Design review of the part built by this model. Coordinates are the model's own, in mm. A direction names the side the tool comes from. Coordinates: 2 decimals unless noted, no trailing zeros. Loops run counter-clockwise (first coordinate to the right, second up) from the corner with the lowest first, then second, coordinate; pieces in that order, holes last. Notation, with made-up numbers: M 34,61.5 L 85,61.5 A31 ccw 85,87.5 Z; hole C 27,0.5 d4. An arc over 180 degrees is marked long. One line per item, written item: value.
```python
from build123d import *

# Parameters (mm, degrees)
SKETCH1_W           = 220
SKETCH1_H           = 39
BOSS_EXTRUDE1_DEPTH = 3
SKETCH2_W           = 155
SKETCH2_H           = 8
SKETCH2_W_2         = 80
SKETCH2_H_2         = 3
SKETCH2_R           = 1.5
CUT_EXTRUDE2_DEPTH  = 3


with BuildPart() as part:
    # Sketch1 → Boss-Extrude1 (new body)
    with BuildSketch(Plane(origin=(0, 0, 0), x_dir=(1, 0, 0), z_dir=(0, 1, 0))):
        Rectangle(SKETCH1_W, SKETCH1_H)
    extrude(amount=BOSS_EXTRUDE1_DEPTH)

    # Sketch2 → Cut-Extrude2 (cut)
    with BuildSketch(Plane.XZ):
        Polygon((-77, 16.5), (-80, 16.5), (-80, 13.5), (-81.25, 13.5), (-81.25, 10.5), (-80, 10.5), (-80, 8.5), (-77, 8.5), (-77, 10.5), (-75.75, 10.5), (-75.75, 13.5), (-77, 13.5), align=None)
        Polygon((-110, 16.5), (-80, 16.5), (-77, 16.5), (-70, 16.5), (-70, 19.5), (-110, 19.5), align=None)
        with Locations((-17.5, -15.5)):
            Rectangle(SKETCH2_W, SKETCH2_H)
        Polygon((110, 19.5), (75, 19.5), (75, 16.5), (75, -13), (75, -19.5), (110, -19.5), align=None)
        Polygon((75, 16.5), (75, 19.5), (30, 19.5), (30, 16.5), (37, 16.5), (40, 16.5), align=None)
        Polygon((40, 13.5), (40, 16.5), (37, 16.5), (37, 13.5), (35.75, 13.5), (35.75, 10.5), (37, 10.5), (37, 8.5), (40, 8.5), (40, 10.5), (41.25, 10.5), (41.25, 13.5), align=None)
        with Locations((-20, 18)):
            Rectangle(SKETCH2_W_2, SKETCH2_H_2)
        with Locations(Location((-102.5, -17, 0), (0, 0, 270))):
            Circle(SKETCH2_R)
        with Locations(Location((67.5, -17, 0), (0, 0, 270))):
            Circle(SKETCH2_R)
    extrude(amount=-CUT_EXTRUDE2_DEPTH, mode=Mode.SUBTRACT)


solid = part.part
```
(1) Tool access review of faces 1 (the flat face through (-19, 1, -11.5)), 2 (the flat face through (30, 1, 18)), 3 (the flat face through (-81.25, 1, 12)), 4 (the flat face through (40, 1, 15)), 5 (the flat face through (-70, 1, 18)): name each direction out of +Z, -Z, +X, -X, +Y, -Y from which nothing blocks a thin tool from reaching the whole face with its end or side.
Reply:
face 1: -Z, +Y, -Y
face 2: +Z, +X, +Y, -Y
face 3: +Y, -Y
face 4: +Z, +Y, -Y
face 5: +Z, -X, +Y, -Y
(2) Insertion check: pin 1 (1.4 mm diameter, centred on x = -80.5, y = 1.5, fed in from -Z); pin 2 (0.6 mm diameter, centred on x = -76, y = 1.5, fed in from +Z). Each pin has a flat end and moves straight along its axis. Give the tip position at first contact, or say it passes through.
Reply:
pin 1: stops at z = -11.5
pin 2: stops at z = 16.5
(3) We need section B-B on x = -9. State the section outline as (y, z) points, then the cut area to 3 significant figures.
Reply:
outline: M 0,-11.5 L 3,-11.5 L 3,16.5 L 0,16.5 Z
area: 84.0 mm2
(4) To check wall thickness, follow line 1 along X through (y, z) = (1.3, -17); line 2 along X through (y, z) = (2.8, 11.5); line 3 along Z through (x, y) = (-102.5, 0.85). State the ranges of each line that lie inside material, in increasing order. Write a range as [from, to].
Reply:
line 1: x = [-110, -104], [-101, -95], [60, 66], [69, 75]
line 2: x = [-110, -81.25], [-75.75, 35.75], [41.25, 75]
line 3: z = [-19.5, -18.5], [-15.5, 16.5]
(5) We need section A-A on y = 2.2. State how many separate pieces and enclosed holes the cut face has, then the cut area to 3 significant figures.
Reply:
separate pieces: 1
enclosed holes: 2
area: 5,400 mm2
(6) Mouldability with a two-part tool opening along Z and no side actions: class faces 6 (the cylindrical face through (-101, 1, -17)), 7 (the flat face through (-19, 0, 0)), 8 (the flat face through (33, 1, 16.5)) as released by +Z, released by -Z, zero draft, split by the parting line, or undercut.
Reply:
face 6: undercut
face 7: zero draft
face 8: released by +Z
